```python
from build123d import *

# Parameters (mm, degrees)
SKETCH_1_W          = 42.3
SKETCH_1_H          = 42.3
EXTRUDE_1_DEPTH     = 3
SKETCH_2_R          = 1.5
CUT_EXTRUDE_1_DEPTH = 3
SKETCH_3_R          = 12.5
CUT_EXTRUDE_2_DEPTH = 3
EXTRUDE_2_DEPTH     = 48
SKETCH_5_W          = 5
SKETCH_5_H          = 47.3
EXTRUDE_3_DEPTH     = 10
SKETCH_6_W          = 5
SKETCH_6_H          = 47.3
EXTRUDE_4_DEPTH     = 10
SKETCH_7_R          = 1.5
CUT_EXTRUDE_3_DEPTH = 10
SKETCH_8_W          = 44.7
SKETCH_8_H          = 45
CUT_EXTRUDE_4_DEPTH = 42.3
SKETCH_10_W         = 10
SKETCH_10_H         = 13
SKETCH_10_H_2       = 10
CUT_EXTRUDE_5_DEPTH = 10


with BuildPart() as part:
    # 草图1 → 凸台-拉伸1 (new body)
    with BuildSketch(Plane.XY):
        Rectangle(SKETCH_1_W, SKETCH_1_H)
    extrude(amount=EXTRUDE_1_DEPTH)

    # 草图2 → 切除-拉伸1 (cut)
    with BuildSketch(Plane.XY.offset(3)):
        with Locations((-15.5, 15.5)):
            Circle(SKETCH_2_R)
        with Locations((15.5, 15.5)):
            Circle(SKETCH_2_R)
        with Locations((15.5, -15.5)):
            Circle(SKETCH_2_R)
        with Locations((-15.5, -15.5)):
            Circle(SKETCH_2_R)
    extrude(amount=-CUT_EXTRUDE_1_DEPTH, mode=Mode.SUBTRACT)

    # 草图3 → 切除-拉伸2 (cut)
    with BuildSketch(Plane.XY.offset(3)):
        Circle(SKETCH_3_R)
    extrude(amount=-CUT_EXTRUDE_2_DEPTH, mode=Mode.SUBTRACT)

    # 草图4 → 凸台-拉伸2 (add)
    with BuildSketch(Plane.XY.offset(3)):
        Polygon((-26.15, -26.15), (26.15, -26.15), (26.15, 21.15), (21.15, 21.15), (21.15, -21.15), (-21.15, -21.15), (-21.15, 21.15), (-26.15, 21.15), align=None)
    extrude(amount=-EXTRUDE_2_DEPTH)

    # 草图5 → 凸台-拉伸3 (add)
    with BuildSketch(Plane.ZY.offset(26.15)):
        with Locations((-4.5, -2.5)):
            Rectangle(SKETCH_5_W, SKETCH_5_H)
    extrude(amount=EXTRUDE_3_DEPTH)

    # 草图6 → 凸台-拉伸4 (add)
    with BuildSketch(Plane(origin=(26.15, 0, 0), x_dir=(0, 0, -1), z_dir=(1, 0, 0))):
        with Locations((4.5, -2.5)):
            Rectangle(SKETCH_6_W, SKETCH_6_H)
    extrude(amount=EXTRUDE_4_DEPTH)

    # 草图7 → 切除-拉伸3 (cut)
    with BuildSketch(Plane.XY.offset(3)):
        with Locations((-33.15, -13.15)):
            Circle(SKETCH_7_R)
        with Locations((-33.15, 5.15)):
            Circle(SKETCH_7_R)
        with Locations(Location((33.15, -13.15, 0), (0, 0, 180))):
            Circle(SKETCH_7_R)
        with Locations(Location((33.15, 5.15, 0), (0, 0, 180))):
            Circle(SKETCH_7_R)
    extrude(amount=-CUT_EXTRUDE_3_DEPTH, mode=Mode.SUBTRACT)

    # 草图8 → 切除-拉伸4 (cut)
    with BuildSketch(Plane(origin=(0, 21.15, 0), x_dir=(1, 0, 0), z_dir=(0, 1, 0))):
        with Locations((0, 22.5)):
            Rectangle(SKETCH_8_W, SKETCH_8_H)
    extrude(amount=-CUT_EXTRUDE_4_DEPTH, mode=Mode.SUBTRACT)

    # 草图10 → 切除-拉伸5 (cut)
    with BuildSketch(Plane.XY.offset(-2)):
        with Locations((-31.15, 14.65)):
            Rectangle(SKETCH_10_W, SKETCH_10_H)
        with Locations((31.15, 14.65)):
            Rectangle(SKETCH_10_W, SKETCH_10_H)
        with Locations((-31.15, -21.15)):
            Rectangle(SKETCH_10_W, SKETCH_10_H_2)
        with Locations((31.15, -21.15)):
            Rectangle(SKETCH_10_W, SKETCH_10_H_2)
    extrude(amount=-CUT_EXTRUDE_5_DEPTH, mode=Mode.SUBTRACT)


solid = part.part
```
Can you work these out from the model? Positions are in its coordinate system, mm. A direction names the side the tool comes from. Coordinates: 2 decimals unless noted, no trailing zeros. Loops run counter-clockwise (first coordinate to the right, second up) from the corner with the lowest first, then second, coordinate; pieces in that order, holes last. Notation, with made-up numbers: (3.25, -26.75) -> (61.25, -26.75) arc R7 ccw to (61.25, -22.75) -> close; hole circle Ø1 at (76, 37). An arc over 180 degrees is marked (long way). Answer as a JSON object with one key per item and string values.
1) For faces 1 (the face through (31, -4, -7)), 2 (the face through (22.35, 0, -22)), 3 (the face through (-31, -4, -7)), which set-ups out of +Z, -Z, +X, -X, +Y, -Y let a thin tool reach every point of the face, with its end or its side?
Results:
{"face 1": "-Z, +X, +Y, -Y", "face 2": "-Z, +Y", "face 3": "-Z, -X, +Y, -Y"}
2) Imagine slicing it at C-C (y = 0). Please give me the cut outline in (x, z), then the cut area to 3 significant figures.
Results:
{"outline": "(-36.15, -7) -> (-26.15, -7) -> (-26.15, -45) -> (-22.35, -45) -> (-22.35, 0) -> (-12.5, 0) -> (-12.5, 3) -> (-26.15, 3) -> (-26.15, -2) -> (-36.15, -2) -> close; (12.5, 0) -> (22.35, 0) -> (22.35, -45) -> (26.15, -45) -> (26.15, -7) -> (36.15, -7) -> (36.15, -2) -> (26.15, -2) -> (26.15, 3) -> (12.5, 3) -> close", "area": "524 mm^2"}
3) Imagine slicing it at A-A (x = 15.5). Please give me the cut outline in (y, z).
Results:
{"outline": "(-26.15, -45) -> (-21.15, -45) -> (-21.15, 0) -> (-17, 0) -> (-17, 3) -> (-26.15, 3) -> close; (-14, 0) -> (14, 0) -> (14, 3) -> (-14, 3) -> close; (17, 0) -> (21.15, 0) -> (21.15, 3) -> (17, 3) -> close"}
4) For P1, Ø1, axis at x = 13, z = -38, coming from the +Y side; P2, Ø2.5, axis at x = 32, z = -3.5, coming from the -Y side; P3, Ø3, axis at x = -32.5, y = -6, coming from the +Z side; P4, Ø10, axis at x = 19, y = 14.5, coming from the -Z side, each with a flat end and sliding along its axis, tell me the tip position at first contact or that it passes through.
Results:
{"P1": "stops at y = -21.15", "P2": "stops at y = -16.15", "P3": "stops at z = -2", "P4": "stops at z = -45"}
5) Imagine slicing it at B-B (z = -4.5). Please give me the cut outline in (x, y).
Results:
{"outline": "(-36.15, -16.15) -> (-26.15, -16.15) -> (-26.15, -26.15) -> (26.15, -26.15) -> (26.15, -16.15) -> (36.15, -16.15) -> (36.15, 8.15) -> (26.15, 8.15) -> (26.15, 21.15) -> (22.35, 21.15) -> (22.35, -21.15) -> (-22.35, -21.15) -> (-22.35, 21.15) -> (-26.15, 21.15) -> (-26.15, 8.15) -> (-36.15, 8.15) -> close; hole circle Ø3 at (-33.15, -13.15); hole circle Ø3 at (-33.15, 5.15); hole circle Ø3 at (33.15, -13.15); hole circle Ø3 at (33.15, 5.15)"}
6) If I drill on line 1 (X direction, y = -13, z = -3); line 2 (Y direction, x = -33.15, z = -5.2); line 3 (Y direction, x = 15.5, z = 1.4), over which ranges is the centre line in solid material (lowest first)?
Results:
{"line 1": "x = -36.15 to -34.64, -31.66 to -22.35, 22.35 to 31.66, 34.64 to 36.15", "line 2": "y = -16.15 to -14.65, -11.65 to 3.65, 6.65 to 8.15", "line 3": "y = -26.15 to -17, -14 to 14, 17 to 21.15"}
7) Imagine slicing it at D-D (x = 0). Please give me the cut outline in (y, z).
Results:
{"outline": "(-26.15, -45) -> (-21.15, -45) -> (-21.15, 0) -> (-12.5, 0) -> (-12.5, 3) -> (-26.15, 3) -> close; (12.5, 0) -> (21.15, 0) -> (21.15, 3) -> (12.5, 3) -> close"}
8) Thinking about a two-plate mould opening in Y: for faces 4 (the face through (-31, -4, -2)), 5 (the face through (14, 15.57, 1.52)), 6 (the face through (31, 8.15, -4)), which applies, pulls with the +Y half, pulls with the -Y half, needs draft (parallel to the pull), parting line crosses it, or undercut?
Results:
{"face 4": "needs draft", "face 5": "undercut", "face 6": "pulls with the +Y half"}
